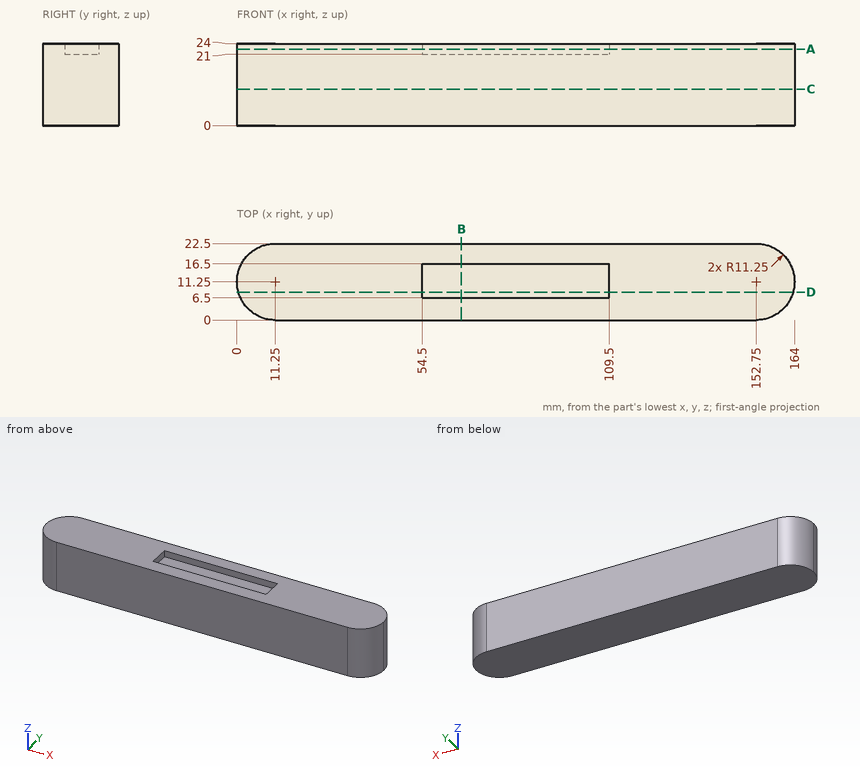
The figure shows three views and two pictorial views of one solid part (mm, origin at its lowest corner). Answer the questions. Give positions to 0.01 mm unless a question says otherwise; leave off trailing zeros. Write each loop counter-clockwise with the first axis right and the second up, starting at its lowest first coordinate (ties: lowest second). Pieces come first, ordered by that corner, then holes. Notation, with made-up numbers: (58, -8) -> (87, -8) arc R25 ccw to (87, 10) -> close; hole circle Ø1 at (58, -4). An arc over 180 degrees is marked (long way). Answer as a JSON object with one key per item and string values.
1) Section A-A on z = 22.5 is taken. Write down the section's boundary in (x, y), then the cut area to 3 significant figures.
Findings below:
{"outline": "(11.25, 0) -> (152.75, 0) arc R11.25 ccw to (152.75, 22.5) -> (11.25, 22.5) arc R11.25 ccw to start; hole (54.5, 6.5) -> (109.5, 6.5) -> (109.5, 16.5) -> (54.5, 16.5) -> close", "area": "3,030 mm^2"}
2) Section B-B on x = 66 is taken. Write down the section's boundary in (y, z), then the cut area to 3 significant figures.
Findings below:
{"outline": "(0, 0) -> (22.5, 0) -> (22.5, 24) -> (16.5, 24) -> (16.5, 21) -> (6.5, 21) -> (6.5, 24) -> (0, 24) -> close", "area": "510 mm^2"}
3) Flat-ended cylindrical pins translate along their axes: pin 1 Ø4 at (y, z) = (18.5, 10) entering from +X; pin 2 Ø4 at (y, z) = (9, 20.5) entering from +X; pin 3 Ø2 at (y, z) = (6.5, 2.5) entering from -X. Find the tip coordinate at first contact, or state that the pin passes through.
Findings below:
{"pin 1": "stops at x = 162.7", "pin 2": "stops at x = 164", "pin 3": "stops at x = 0.64"}
4) Section C-C on z = 10.75 is taken. Write down the section's boundary in (x, y), then the cut area to 3 significant figures.
Findings below:
{"outline": "(11.25, 0) -> (152.75, 0) arc R11.25 ccw to (152.75, 22.5) -> (11.25, 22.5) arc R11.25 ccw to start", "area": "3,580 mm^2"}
5) Straight lines are drawn through the part: probe 1 along X at (y, z) = (10.5, 21.25); probe 2 along Y at (x, z) = (81, 23); probe 3 along X at (y, z) = (8.75, 23). For each, find the intervals that lie inside material, in ascending order. Write a range as from..to.
Findings below:
{"probe 1": "x = 0.03..54.5, 109.5..163.97", "probe 2": "y = 0..6.5, 16.5..22.5", "probe 3": "x = 0.28..54.5, 109.5..163.72"}
6) Section D-D on y = 8.25 is taken. Write down the section's boundary in (x, z).
Findings below:
{"outline": "(0.41, 0) -> (163.59, 0) -> (163.59, 24) -> (109.5, 24) -> (109.5, 21) -> (54.5, 21) -> (54.5, 24) -> (0.41, 24) -> close"}
